Drawing for the job (mm, zero at the part's lowest x, y, z). A direction names the side the tool comes from. Coordinates: 2 decimals unless noted, no trailing zeros. Loops run counter-clockwise (first coordinate to the right, second up) from the corner with the lowest first, then second, coordinate; pieces in that order, holes last. Notation, with made-up numbers: (31, 62) -> (49, 62) arc R10 cw to (49, 73) -> close; hole circle Ø11 at (-12, 5.25). An arc over 180 degrees is marked (long way). Write item = value, one per line. Start each with the question number.
(1) Band-saw the part on A-A (x = 83.5). Count the separate pieces of the cut face and the enclosed holes in it, and give its area (3 significant figures).
(2) Band-saw the part on B-B (y = 25). Write the cut outline in (x, z), and give its area (3 significant figures).
(3) Band-saw the part on C-C (z = 16.75). Write the cut outline in (x, y) (1 decimal), and give its area (3 significant figures).
(4) Flat gauge pins, fed straight in: P1, Ø17, axis at x = 72.97, y = 69.81, coming from the -Z side; P2, Ø6, axis at x = 78, z = 6.5, coming from the -Y side; P3, Ø7, axis at y = 73.5, z = 20.5, coming from the -X side (1 decimal); P4, Ø5, axis at x = 12, z = 7, coming from the +Y side. Where does each tip first touch, or does it go through?
(5) Drill centre lines: line 1 (Z direction, x = 93, y = 83.5); line 2 (Y direction, x = 66, z = 6) (1 decimal); line 3 (Y direction, x = 42, z = 12.5). Where is each one in solid material? Low to high. Write a range as from..to.
(6) Pull direction Z, two halves, no side cores. Call the marked faces 4, 5 and 6: +Z half, -Z half, draft (parallel to the pull), parting line (faces both ways), or undercut.
(7) Band-saw the part on D-D (x = 13). Write the cut outline in (y, z) (1 decimal).
(8) Tool access for the marked faces 1, 2 and 3: list every direction of +Z, -Z, +X, -X, +Y, -Y with a clear straight run to the whole face (end or side of a thin tool).
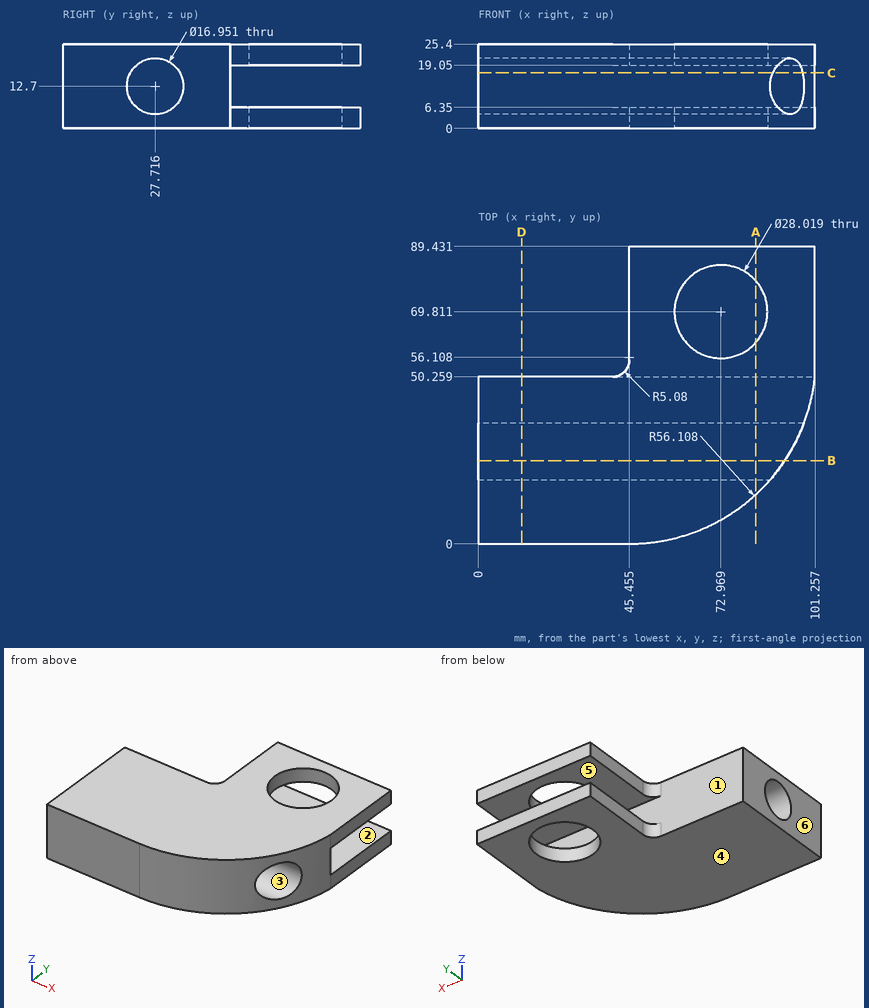
Findings below:
q1.separate_pieces = 3
q1.enclosed_holes = 1
q1.area = 936 mm²
q2.outline = (0, 0) -> (92.15, 0) -> (92.15, 4.67) -> (0, 4.67) -> close; (0, 20.73) -> (92.15, 20.73) -> (92.15, 25.4) -> (0, 25.4) -> close
q2.area = 861 mm²
q3.outline = (0, 0) -> (45.5, 0) arc R56.1 ccw to (88.6, 20.3) -> (0, 20.3) -> close; (0, 35.2) -> (97.5, 35.2) arc R56.1 ccw to (101.3, 50.3) -> (0, 50.3) -> close
q3.area = 3,040 mm²
q4.P1 = through
q4.P2 = 8.41
q4.P3 = 45.5
q4.P4 = 50.26
q5.line_1 = 0..6.35, 19.05..25.4
q5.line_2 = 3.9..22.5, 32.9..57.7, 82..89.4
q5.line_3 = 0..19.24, 36.19..50.26
q6.face_4 = -Z half
q6.face_5 = undercut
q6.face_6 = draft
q7.outline = (0, 0) -> (50.3, 0) -> (50.3, 25.4) -> (0, 25.4) -> close; hole circle Ø17 at (27.7, 12.7)
q8.face_1 = -X, +Y
q8.face_2 = +X, -X, +Y
q8.face_3 = +X, -X
